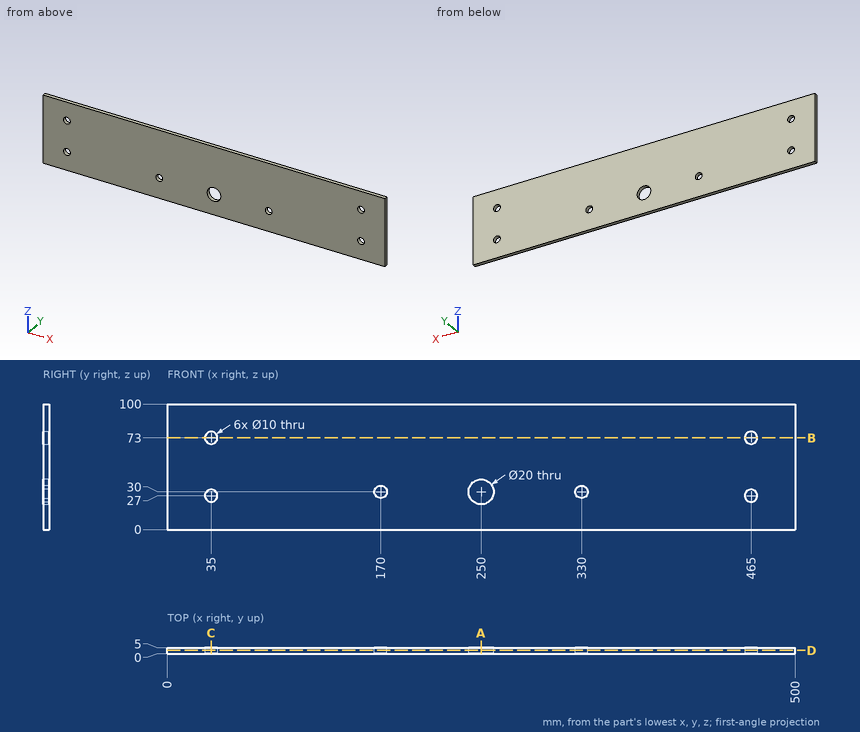
Source: three-view drawing plus pictorial views. Frame: mm from the lowest corner of the part. Round coordinates to 2 decimals unless told otherwise and drop trailing zeros. Loops run counter-clockwise (first coordinate to the right, second up) from the corner with the lowest first, then second, coordinate; pieces in that order, holes last.
1. Section query B-B on z = 73. Output: boundary loops of the cut face in (x, y), and give its area (3 significant figures).
2. Contact query for flat-ended pins moving along their axis: pin 1 (13 mm diameter, centred on x = 170, z = 30, fed in from +Y); pin 2 (8 mm diameter, centred on x = 465, z = 27, fed in from +Y). Output: stop coordinate, or through.
3. Ray query, L1, parallel to Z at x = 465, y = 1.6; L2, parallel to X at y = 2.5, z = 27; L3, parallel to Z at x = 245, y = 3.7. Return the intervals inside material, ascending.
4. Section query A-A on x = 250. Output: boundary loops of the cut face in (y, z), and give its area (3 significant figures).
5. Section query D-D on y = 2.65. Output: boundary loops of the cut face in (x, z), and give its area (3 significant figures).
6. Section query C-C on x = 35. Output: boundary loops of the cut face in (y, z), and give its area (3 significant figures).
Answers below:
1. outline: (0, 0) - (30, 0) - (30, 5) - (0, 5) - close; (40, 0) - (460, 0) - (460, 5) - (40, 5) - close; (470, 0) - (500, 0) - (500, 5) - (470, 5) - close
1. area: 2,400 mm2
2. pin 1: stops at y = 5
2. pin 2: passes through
3. L1: z = 0 to 22, 32 to 68, 78 to 100
3. L2: x = 0 to 30, 40 to 166, 174 to 240.46, 259.54 to 326, 334 to 460, 470 to 500
3. L3: z = 0 to 21.34, 38.66 to 100
4. outline: (0, 0) - (5, 0) - (5, 20) - (0, 20) - close; (0, 40) - (5, 40) - (5, 100) - (0, 100) - close
4. area: 400 mm2
5. outline: (0, 0) - (500, 0) - (500, 100) - (0, 100) - close; hole circle Ø10 at (35, 27); hole circle Ø10 at (35, 73); hole circle Ø10 at (170, 30); hole circle Ø20 at (250, 30); hole circle Ø10 at (330, 30); hole circle Ø10 at (465, 27); hole circle Ø10 at (465, 73)
5. area: 49,200 mm2
6. outline: (0, 0) - (5, 0) - (5, 22) - (0, 22) - close; (0, 32) - (5, 32) - (5, 68) - (0, 68) - close; (0, 78) - (5, 78) - (5, 100) - (0, 100) - close
6. area: 400 mm2
